Part model, mm, in its own coordinate system. A direction names the side the tool comes from. Give positions to 0.01 mm unless a question says otherwise; leave off trailing zeros. Write each loop counter-clockwise with the first axis right and the second up, starting at its lowest first coordinate (ties: lowest second). Pieces come first, ordered by that corner, then holes. Notation, with made-up numbers: (-8, 80) - (12, 80) arc R26 ccw to (12, 112) - close; hole circle Ø10 at (64, 66.25). An arc over 180 degrees is marked (long way). Answer in a Markdown table with one row per item. Add a question column.
1. Band-saw the part on B-B on x = 12.5. Write the cut outline in (y, z), plus the area to 3 significant figures.
2. Band-saw the part on D-D on z = 6. Write the cut outline in (x, y).
3. Pull direction Y, two halves, no side cores. Call faces 4 (the cylindrical face through (-59, -15.7, 21.5)), 5 (the cylindrical face through (48.797, -62.859, 18.252)), 6 (the flat face through (50, -32, 18)): released by +Y, released by -Y, zero draft, split by the parting line, or undercut.
4. Band-saw the part on A-A on y = -37.5. Write the cut outline in (x, z).
5. Band-saw the part on C-C on z = 21.5. Write the cut outline in (x, y).
6. Which spindle directions (+Z, -Z, +X, -X, +Y, -Y) get a long thin tool onto all of the face, cutting with end or side? Do faces 1 (the flat face through (-52, -13, 24)), 2 (the flat face through (-25.1, -25, 18)), 3 (the cylindrical face through (-63.859, -51.203, 9.367)). Say none if no direction does.
7. Probe line 1 along X through (y, z) = (-15, 32.75); line 2 along X through (y, z) = (-15, 5); line 3 along X through (y, z) = (-59.5, 13.5). List the from-to ranges inside material, lowest first.
8. Drop flat-ended pins along their axis: pin 1 Ø3 at (x, y) = (37.55, -15) entering from +Z; pin 2 Ø4 at (x, z) = (13, 21.5) entering from +Y; pin 3 Ø11 at (y, z) = (-22, 11) entering from -X; pin 4 Ø9 at (x, y) = (-54.05, -15) entering from -Z. Give the stop position or say it passes through.
Autodesk Inventor part; units mm, degrees
ref_plane "YZ Plane" through (0, 0, 0) normal (1, 0, 0) x (0, 1, 0)
ref_plane "XZ Plane" through (0, 0, 0) normal (0, 1, 0) x (-1, 0, 0)
ref_plane "XY Plane" through (0, 0, 0) normal (0, 0, 1) x (1, 0, 0)
sketch "Sketch1" plane through (0, 0, 0) normal (0, 0, 1) x (1, 0, 0)
  line L0 (-50, -64) -> (50, -64)
  line L1 (50, -64) -> (50, 0)
  line L2 (50, 0) -> (-50, 0)
  line L3 (-50, 0) -> (-50, -64)
  line L4 (-50, -64) -> (50, 0) construction
  line L5 (50, -64) -> (-50, 0) construction
  line L6 (-25.1, -50) -> (25.1, -50)
  line L7 (25.1, -50) -> (25.1, 0)
  line L8 (25.1, 0) -> (-25.1, 0)
  line L9 (-25.1, 0) -> (-25.1, -50)
  line L10 (-25.1, -50) -> (25.1, 0) construction
  line L11 (25.1, -50) -> (-25.1, 0) construction
  point P0 (0, 0)
  point P1 (0, -32)
  point P2 (0, 0)
  point P3 (0, -25)
  point P4 (-25.1, 0)
  dimension "d0" = 100
  dimension "d1" = 64
  dimension "d2" = 50.2
  dimension "d3" = 50
extrude "Extrusion1" add sketch "Sketch1" along normal blind 36 contours L3 L2 L9 L6 L7 L1 L0
sketch "Sketch2" plane through (0, 0, 0) normal (0, 0, -1) x (-1, 0, 0)
  line L0 (-50, 0) -> (-25.1, 0)
  line L1 (-25.1, 0) -> (-25.1, -50)
  line L2 (-25.1, -50) -> (25.1, -50)
  line L3 (25.1, -50) -> (25.1, 0)
  line L4 (25.1, 0) -> (50, 0)
  line L5 (50, 0) -> (50, -64)
  line L6 (50, -64) -> (-50, -64)
  line L7 (-50, -64) -> (-50, 0)
  line L8 (25.1, 0) -> (50, 0)
  line L9 (50, 0) -> (50, -50)
  line L10 (50, -50) -> (25.1, -50)
  line L11 (25.1, -50) -> (25.1, 0)
  point P0 (0, 0)
  point P1 (25.1, -50)
extrude "Extrusion2" cut sketch "Sketch2" against normal blind 19 contours L3 L4 L5 L10
sketch "Sketch3" plane through (-50, -64, 0) normal (-1, 0, 0) x (0, 0, 1)
  line L0 (19, 64) -> (19, 14)
  line L1 (19, 14) -> (0, 14)
  line L2 (0, 14) -> (0, 0)
  line L3 (0, 0) -> (36, 0)
  line L4 (36, 64) -> (36, 0)
  line L5 (19, 64) -> (36, 64)
  point P0 (0, 64)
extrude "Extrusion3" add sketch "Sketch3" along normal blind 15
sketch "Sketch4" plane through (0, 0, 0) normal (0, 0, -1) x (-1, 0, 0)
  line L0 (-25.1, -50) -> (65, -50)
  line L1 (-25.1, 0) -> (-25.1, -50)
  line L2 (-50, 0) -> (-25.1, 0)
  line L3 (-50, -64) -> (-50, 0)
  line L4 (-50, -64) -> (65, -64)
  line L5 (65, -50) -> (65, -64)
  line L6 (-50, 0) -> (-25.1, 0)
  point P0 (0, 0)
  point P1 (-37.55, -15)
  point P2 (-37.55, 0)
  point P3 (-37.55, 0)
  dimension "d10" = 15
hole "Hole1" at (37.55, -15, 0) direction (0, 0, 1) diameter 5.2 end through all counterbore diameter 10 counterbore depth 14
sketch "Sketch5" plane through (0, 0, 19) normal (0, 0, -1) x (-1, 0, 0)
  line L0 (25.1, 0) -> (65, 0)
  line L1 (25.1, -50) -> (25.1, 0)
  line L2 (65, -50) -> (25.1, -50)
  line L3 (65, 0) -> (65, -50)
  line L4 (36.05, -15) -> (54.05, -15) construction
  point P0 (0, 0)
  point P1 (45.05, 0)
  point P2 (45.05, -15)
  dimension "d18" = 18
  dimension "d19" = 15
hole "Hole2" at (-54.05, -15, 19) direction (0, 0, 1) diameter 5.2 end through all counterbore diameter 10 counterbore depth 5
sketch "Sketch6" plane through (0, 0, 19) normal (0, 0, -1) x (-1, 0, 0)
  circle A0 centre (54.05, -15) radius 5
  line L0 (25.1, 0) -> (65, 0)
  line L1 (25.1, -50) -> (25.1, 0)
  line L2 (65, -50) -> (25.1, -50)
  line L3 (65, 0) -> (65, -50)
  line L4 (25.1, 0) -> (39.1, 0)
  line L5 (39.1, 0) -> (39.1, -50)
  line L6 (39.1, -50) -> (25.1, -50)
  line L7 (25.1, -50) -> (25.1, 0)
  point P0 (0, 0)
  point P1 (39.1, 0)
  dimension "d27" = 14
extrude "Extrusion4" add sketch "Sketch6" along normal up to surface (19 mm away) contours L0 L5 L2 L1
sketch "Sketch7" plane through (-39.1, -50, 19) normal (-1, 0, 0) x (0, 0, 1)
  circle A0 centre (-5.5, 37.5) radius 2.067
  circle A1 centre (-5.5, 12.5) radius 2.067
  point P0 (-19, 50)
hole "Hole3" at (-39.1, -12.5, 13.5) at (-39.1, -37.5, 13.5) direction (1, 0, 0) diameter 5.2 depth 14
sketch "Sketch8" plane through (50, -64, 0) normal (0, -1, 0) x (1, 0, 0)
  circle A0 centre (-37.5, 13.5) radius 2.067
  circle A1 centre (-62.5, 13.5) radius 2.067
  point P0 (-50, 0)
hole "Hole4" at (12.5, -64, 13.5) at (-12.5, -64, 13.5) direction (0, 1, 0) diameter 5.2 end through all
fillet "Fillet1" radius 4 7 edges at (50, 0, 18) (50, -64, 18) (-65, -64, 18) (-65, 0, 27.5) (-39.1, -50, 9.5) (-39.1, 0, 9.5) (-65, -50, 9.5)
properties part number "lift_encoder_frame" material "ABS Plastic"
Values:
| question | item | result |
|---|---|---|
| 1 | outline | (-64, 0) - (-50, 0) - (-50, 10.9) - (-64, 10.9) - close; (-64, 16.1) - (-50, 16.1) - (-50, 36) - (-64, 36) - close |
| 1 | area | 431 mm² |
| 2 | outline | (-65, -60) arc R4 ccw to (-61, -64) - (46, -64) arc R4 ccw to (50, -60) - (50, -4) arc R4 ccw to (46, 0) - (25.1, 0) - (25.1, -50) - (-25.1, -50) - (-25.1, 0) - (-35.1, 0) arc R4 ccw to (-39.1, -4) - (-39.1, -46) arc R4 cw to (-43.1, -50) - (-61, -50) arc R4 ccw to (-65, -54) - close; hole circle Ø10 at (37.55, -15) |
| 3 | face 4 | undercut |
| 3 | face 5 | released by -Y |
| 3 | face 6 | zero draft |
| 4 | outline | (-65, 19) - (-39.1, 19) - (-39.1, 16.1) - (-25.1, 16.1) - (-25.1, 36) - (-65, 36) - close; (-39.1, 0) - (-25.1, 0) - (-25.1, 10.9) - (-39.1, 10.9) - close; (25.1, 0) - (50, 0) - (50, 36) - (25.1, 36) - close |
| 5 | outline | (-65, -60) arc R4 ccw to (-61, -64) - (46, -64) arc R4 ccw to (50, -60) - (50, -4) arc R4 ccw to (46, 0) - (25.1, 0) - (25.1, -50) - (-25.1, -50) - (-25.1, 0) - (-61, 0) arc R4 ccw to (-65, -4) - close; hole circle Ø10 at (-54.05, -15); hole circle Ø5.2 at (37.55, -15) |
| 6 | face 1 | -Z |
| 6 | face 2 | +Z, -Z, +Y |
| 6 | face 3 | -Z, -X, +Y |
| 7 | line 1 | x = -65 to -56.65, -51.45 to -25.1, 25.1 to 34.95, 40.15 to 50 |
| 7 | line 2 | x = -39.1 to -25.1, 25.1 to 32.55, 42.55 to 50 |
| 7 | line 3 | x = -65 to -15.1, -9.9 to 9.9, 15.1 to 50 |
| 8 | pin 1 | passes through |
| 8 | pin 2 | stops at y = -50 |
| 8 | pin 3 | stops at x = -39.1 |
| 8 | pin 4 | stops at z = 24 |
